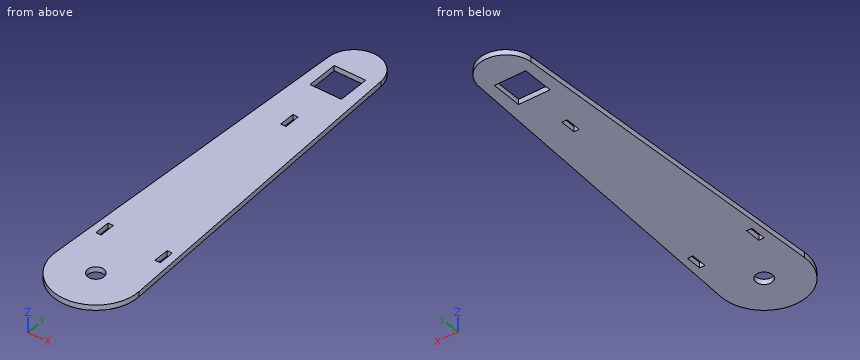
from build123d import *

# Parameters (mm, degrees)
SKETCH1_R           = 4.953
SKETCH1_W           = 3.175
SKETCH1_H           = 9.525
SKETCH1_W_2         = 19.05
SKETCH1_H_2         = 19.05
BOSS_EXTRUDE1_DEPTH = 3.175


with BuildPart() as part:
    # Sketch1 → Boss-Extrude1 (new body)
    with BuildSketch(Plane.XY):
        with BuildLine():
            Line((-25.372181386, 1.188449288), (-15.875, 203.943595206))
            ThreePointArc((-15.875, 203.943595206), (0, 219.092405697), (15.875, 203.943595206))
            Line((15.875, 203.943595206), (25.372181386, 1.188449288))
            ThreePointArc((25.372181386, 1.188449288), (0, -25.4), (-25.372181386, 1.188449288))
        make_face()
        Circle(SKETCH1_R, mode=Mode.SUBTRACT)
        with Locations((-17.9197, 30.1625)):
            Rectangle(SKETCH1_W, SKETCH1_H, mode=Mode.SUBTRACT)
        with Locations((0, 152.4)):
            Rectangle(SKETCH1_W, SKETCH1_H, mode=Mode.SUBTRACT)
        with Locations((17.9197, 30.1625)):
            Rectangle(SKETCH1_W, SKETCH1_H, mode=Mode.SUBTRACT)
        with Locations((0, 190.5)):
            Rectangle(SKETCH1_W_2, SKETCH1_H_2, mode=Mode.SUBTRACT)
    extrude(amount=BOSS_EXTRUDE1_DEPTH)


solid = part.part
Input: part model. Units: mm. Frame: model coordinates. Give positions to 0.01 mm unless a question says otherwise; leave off trailing zeros. Loops run counter-clockwise (first coordinate to the right, second up) from the corner with the lowest first, then second, coordinate; pieces in that order, holes last. Notation, with made-up numbers: (-24.5, -18) -> (-19.5, -18) arc R20 ccw to (-19.5, 3) -> close; hole circle Ø11 at (64, 0.5). An arc over 180 degrees is marked (long way). Answer as a JSON object with one key per item and string values. Group by question number.
Item 1: Line query: probe 1 along Y at (x, z) = (-0.5, 0.6) (1 decimal); probe 2 along Y at (x, z) = (-4.5, 0.45) (3 decimals); probe 3 along Y at (x, z) = (-9, 0.25) (3 decimals). Output: solid intervals per line, ascending.
Item 2: Cut plane C-C, the plane y = 80.5. Return the cut outline in (x, z) (3 decimals).
Item 3: Cut plane B-B, the plane y = 28. Return the cut outline in (x, z) (3 decimals).
Item 4: Cut plane D-D, the plane y = 140.5. Return the cut outline in (x, z) (3 decimals).
Item 5: Pin query (flat end, axial travel): P1, Ø1.6, axis at y = 153, z = 2, coming from the +X side; P2, Ø1.6, axis at y = 191.5, z = 1, coming from the +X side; P3, Ø1.6, axis at x = 3, z = 1.5, coming from the -Y side. Return the tip coordinate at first contact, or that it passes through.
Item 6: Cut plane A-A, the plane z = 0.8. Return the cut outline in (x, y) (1 decimal), and give its area (3 significant figures).
Checks:
{
 "1": {"probe 1": "y = -25.4 to -4.9, 4.9 to 147.6, 157.2 to 181, 200 to 219.1", "probe 2": "y = -24.998 to -2.069, 2.069 to 180.975, 200.025 to 218.442", "probe 3": "y = -23.752 to 180.975, 200.025 to 216.298"},
 "2": {"outline": "(-21.657, 0) -> (21.657, 0) -> (21.657, 3.175) -> (-21.657, 3.175) -> close"},
 "3": {"outline": "(-24.116, 0) -> (-19.507, 0) -> (-19.507, 3.175) -> (-24.116, 3.175) -> close; (-16.332, 0) -> (16.332, 0) -> (16.332, 3.175) -> (-16.332, 3.175) -> close; (19.507, 0) -> (24.116, 0) -> (24.116, 3.175) -> (19.507, 3.175) -> close"},
 "4": {"outline": "(-18.847, 0) -> (18.847, 0) -> (18.847, 3.175) -> (-18.847, 3.175) -> close"},
 "5": {"P1": "stops at x = 18.3", "P2": "stops at x = 16.5", "P3": "stops at y = -25.3"},
 "6": {"outline": "(-25.4, 1.2) arc R25.4 ccw (long way) to (25.4, 1.2) -> (15.9, 203.9) arc R15.9 ccw to (-15.9, 203.9) -> close; hole (-19.5, 25.4) -> (-16.3, 25.4) -> (-16.3, 34.9) -> (-19.5, 34.9) -> close; hole (-9.5, 181) -> (9.5, 181) -> (9.5, 200) -> (-9.5, 200) -> close; hole circle Ø9.9 at (0, 0); hole (-1.6, 147.6) -> (1.6, 147.6) -> (1.6, 157.2) -> (-1.6, 157.2) -> close; hole (16.3, 25.4) -> (19.5, 25.4) -> (19.5, 34.9) -> (16.3, 34.9) -> close", "area": "9,280 mm²"}
}
